Work out the finished part from the listing and answer in its coordinate system (mm). A direction names the side the tool comes from. Coordinates: 2 decimals unless noted, no trailing zeros. Order: outer loops, then holes, each group sorted by start corner. A loop starts at its lowest first (then second) coordinate and runs counter-clockwise, first axis right, second up. Notation, with made-up numbers: M 78.25,12.5 L 99.25,12.5 A19 cw 99.25,19.5 Z; hole C 51.5,-9.75 d6. An arc over 180 degrees is marked long. Answer in a Markdown table with one row per item. Add a question column.
Item 1: Which of the six approach directions +Z, -Z, +X, -X, +Y, -Y give full straight-line access (tool end or side, diameter ignored) to faces 1 (the face through (0.356, -125.274, 10.334)), 2 (the face through (0, -44, 8.21))?
Item 2: The part is cut by section A-A (x = -5.5). Write down the section's boundary in (y, z), then the cut area to 3 significant figures.
Item 3: Flat-ended cylindrical pins translate along their axes: pin 1 Ø2 at (x, z) = (-12.5, 22) entering from -Y; pin 2 Ø10 at (x, y) = (-5, -46.5) entering from -Z; pin 3 Ø2 at (x, z) = (-0.5, 6.5) entering from -Y. Find the tip coordinate at first contact, or state that the pin passes through.
Item 4: The part is cut by section B-B (y = -86.5). Write down the section's boundary in (x, z).
Item 5: The part is cut by section C-C (z = 4). Write down the section's boundary in (x, y), then the cut area to 3 significant figures.
Item 6: Consider line 1 (Y direction, x = -22.5, z = 6.5); line 2 (Z direction, x = -13, y = -101.5); line 3 (Y direction, x = 7, z = 23.5). Determine where each line is inside the solid, lowest interval first. Write a range as from..to.
from build123d import *

# Parameters (mm, degrees)
F1_DEPTH = 25.4
F2_DEPTH = 25.4


with BuildPart() as f1:
    # F0 (on Right) → F1 (new body)
    with BuildSketch(Plane.YZ):
        Polygon((-133.440181613, 37.7011820674), (-134.0246200562, 12.3990774155), (-116.2741854787, 8.210147731), (-103.3477857709, -1.8578846939), (-63.7195706367, -1.8578846939), (-49.0556843579, 8.210147731), (-39.7747755051, 8.210147731), (-39.7747755051, 33.5487276316), align=None)
    extrude(amount=F1_DEPTH)

    # F2 (add): a face of the model
    f2_faces = [f1.faces().sort_by_distance(p)[0] for p in [
        (0, -86.6234005429, 18.8773491823),
    ]]
    extrude(f2_faces, amount=F2_DEPTH)


solid = f1.part
Reply:
| question | item | result |
|---|---|---|
| 1 | face 1 | -Z, +X, -X, -Y |
| 1 | face 2 | -Z, +X, -X, +Y |
| 2 | outline | M -134.02,12.4 L -116.27,8.21 L -103.35,-1.86 L -63.72,-1.86 L -49.06,8.21 L -39.77,8.21 L -39.77,33.55 L -133.44,37.7 Z |
| 2 | area | 3,080 mm2 |
| 3 | pin 1 | stops at y = -133.83 |
| 3 | pin 2 | stops at z = 6.53 |
| 3 | pin 3 | stops at y = -115.36 |
| 4 | outline | M -25.4,-1.86 L 25.4,-1.86 L 25.4,35.62 L -25.4,35.62 Z |
| 5 | outline | M -25.4,-110.87 L 25.4,-110.87 L 25.4,-55.19 L -25.4,-55.19 Z |
| 5 | area | 2,830 mm2 |
| 6 | line 1 | y = -114.08..-51.55 |
| 6 | line 2 | z = -1.86..36.29 |
| 6 | line 3 | y = -133.77..-39.77 |
